For this review, take the finished solid that the model builds, in its own axes (mm). A direction names the side the tool comes from. Give positions to 0.01 mm unless a question says otherwise; leave off trailing zeros. Loops run counter-clockwise (first coordinate to the right, second up) from the corner with the lowest first, then second, coordinate; pieces in that order, holes last. Notation, with made-up numbers: (-35.75, 29) -> (17.25, 29) arc R28 cw to (17.25, 63) -> close; hole circle Ø8 at (34, 44). An arc over 180 degrees is marked (long way). Write each question's results on one line, items separated by ' | '. Start each with the question number.
```python
from build123d import *

# Parameters (mm, degrees)
SKETCH1_R           = 2.6
BOSS_EXTRUDE1_DEPTH = 5


with BuildPart() as part:
    # Sketch1 → Boss-Extrude1 (new body)
    with BuildSketch(Plane(origin=(0, 0, 0), x_dir=(1, 0, 0), z_dir=(0, 1, 0))):
        with BuildLine():
            Line((0.885, 8.705129235), (0.785, 9.969141137))
            Line((0.785, 9.969141137), (0.5, 10.988630488))
            ThreePointArc((0.5, 10.988630488), (0, 11), (-0.5, 10.988630488))
            Line((-0.5, 10.988630488), (-0.785, 9.969141137))
            Line((-0.785, 9.969141137), (-0.885, 8.705129235))
            ThreePointArc((-0.885, 8.705129235), (-1.368801569, 8.64227298), (-1.848347855, 8.552549924))
            Line((-1.848347855, 8.552549924), (-2.334054665, 9.72379498))
            Line((-2.334054665, 9.72379498), (-2.920145308, 10.605317128))
            ThreePointArc((-2.920145308, 10.605317128), (-3.399186938, 10.461621679), (-3.871201824, 10.296300134))
            Line((-3.871201824, 10.296300134), (-3.827213396, 9.238638299))
            Line((-3.827213396, 9.238638299), (-3.531717889, 8.005589844))
            ThreePointArc((-3.531717889, 8.005589844), (-3.972416873, 7.796307087), (-4.400766544, 7.562787438))
            Line((-4.400766544, 7.562787438), (-5.224635797, 8.526616022))
            Line((-5.224635797, 8.526616022), (-6.054446447, 9.183881436))
            ThreePointArc((-6.054446447, 9.183881436), (-6.465637775, 8.899186938), (-6.863463441, 8.596096183))
            Line((-6.863463441, 8.596096183), (-6.494792479, 7.603793176))
            Line((-6.494792479, 7.603793176), (-5.832726624, 6.522407541))
            ThreePointArc((-5.832726624, 6.522407541), (-6.187184335, 6.187184335), (-6.522407541, 5.832726624))
            Line((-6.522407541, 5.832726624), (-7.603793176, 6.494792479))
            Line((-7.603793176, 6.494792479), (-8.596096183, 6.863463441))
            ThreePointArc((-8.596096183, 6.863463441), (-8.899186938, 6.465637775), (-9.183881436, 6.054446447))
            Line((-9.183881436, 6.054446447), (-8.526616022, 5.224635797))
            Line((-8.526616022, 5.224635797), (-7.562787438, 4.400766544))
            ThreePointArc((-7.562787438, 4.400766544), (-7.796307087, 3.972416873), (-8.005589844, 3.531717889))
            Line((-8.005589844, 3.531717889), (-9.238638299, 3.827213396))
            Line((-9.238638299, 3.827213396), (-10.296300134, 3.871201824))
            ThreePointArc((-10.296300134, 3.871201824), (-10.461621679, 3.399186938), (-10.605317128, 2.920145308))
            Line((-10.605317128, 2.920145308), (-9.72379498, 2.334054665))
            Line((-9.72379498, 2.334054665), (-8.552549924, 1.848347855))
            ThreePointArc((-8.552549924, 1.848347855), (-8.64227298, 1.368801569), (-8.705129235, 0.885))
            Line((-8.705129235, 0.885), (-9.969141137, 0.785))
            Line((-9.969141137, 0.785), (-10.988630488, 0.5))
            ThreePointArc((-10.988630488, 0.5), (-11, 0), (-10.988630488, -0.5))
            Line((-10.988630488, -0.5), (-9.969141137, -0.785))
            Line((-9.969141137, -0.785), (-8.705129235, -0.885))
            ThreePointArc((-8.705129235, -0.885), (-8.64227298, -1.368801569), (-8.552549924, -1.848347855))
            Line((-8.552549924, -1.848347855), (-9.72379498, -2.334054665))
            Line((-9.72379498, -2.334054665), (-10.605317128, -2.920145308))
            ThreePointArc((-10.605317128, -2.920145308), (-10.461621679, -3.399186938), (-10.296300134, -3.871201824))
            Line((-10.296300134, -3.871201824), (-9.238638299, -3.827213396))
            Line((-9.238638299, -3.827213396), (-8.005589844, -3.531717889))
            ThreePointArc((-8.005589844, -3.531717889), (-7.796307087, -3.972416873), (-7.562787438, -4.400766544))
            Line((-7.562787438, -4.400766544), (-8.526616022, -5.224635797))
            Line((-8.526616022, -5.224635797), (-9.183881436, -6.054446447))
            ThreePointArc((-9.183881436, -6.054446447), (-8.899186938, -6.465637775), (-8.596096183, -6.863463441))
            Line((-8.596096183, -6.863463441), (-7.603793176, -6.494792479))
            Line((-7.603793176, -6.494792479), (-6.522407541, -5.832726624))
            ThreePointArc((-6.522407541, -5.832726624), (-6.187184335, -6.187184335), (-5.832726624, -6.522407541))
            Line((-5.832726624, -6.522407541), (-6.494792479, -7.603793176))
            Line((-6.494792479, -7.603793176), (-6.863463441, -8.596096183))
            ThreePointArc((-6.863463441, -8.596096183), (-6.465637775, -8.899186938), (-6.054446447, -9.183881436))
            Line((-6.054446447, -9.183881436), (-5.224635797, -8.526616022))
            Line((-5.224635797, -8.526616022), (-4.400766544, -7.562787438))
            ThreePointArc((-4.400766544, -7.562787438), (-3.972416873, -7.796307087), (-3.531717889, -8.005589844))
            Line((-3.531717889, -8.005589844), (-3.827213396, -9.238638299))
            Line((-3.827213396, -9.238638299), (-3.871201824, -10.296300134))
            ThreePointArc((-3.871201824, -10.296300134), (-3.399186938, -10.461621679), (-2.920145308, -10.605317128))
            Line((-2.920145308, -10.605317128), (-2.334054665, -9.72379498))
            Line((-2.334054665, -9.72379498), (-1.848347855, -8.552549924))
            ThreePointArc((-1.848347855, -8.552549924), (-1.368801569, -8.64227298), (-0.885, -8.705129235))
            Line((-0.885, -8.705129235), (-0.785, -9.969141137))
            Line((-0.785, -9.969141137), (-0.5, -10.988630488))
            ThreePointArc((-0.5, -10.988630488), (0, -11), (0.5, -10.988630488))
            Line((0.5, -10.988630488), (0.785, -9.969141137))
            Line((0.785, -9.969141137), (0.885, -8.705129235))
            ThreePointArc((0.885, -8.705129235), (1.368801569, -8.64227298), (1.848347855, -8.552549924))
            Line((1.848347855, -8.552549924), (2.334054665, -9.72379498))
            Line((2.334054665, -9.72379498), (2.920145308, -10.605317128))
            ThreePointArc((2.920145308, -10.605317128), (3.399186938, -10.461621679), (3.871201824, -10.296300134))
            Line((3.871201824, -10.296300134), (3.827213396, -9.238638299))
            Line((3.827213396, -9.238638299), (3.531717889, -8.005589844))
            ThreePointArc((3.531717889, -8.005589844), (3.972416873, -7.796307087), (4.400766544, -7.562787438))
            Line((4.400766544, -7.562787438), (5.224635797, -8.526616022))
            Line((5.224635797, -8.526616022), (6.054446447, -9.183881436))
            ThreePointArc((6.054446447, -9.183881436), (6.465637775, -8.899186938), (6.863463441, -8.596096183))
            Line((6.863463441, -8.596096183), (6.494792479, -7.603793176))
            Line((6.494792479, -7.603793176), (5.832726624, -6.522407541))
            ThreePointArc((5.832726624, -6.522407541), (6.187184335, -6.187184335), (6.522407541, -5.832726624))
            Line((6.522407541, -5.832726624), (7.603793176, -6.494792479))
            Line((7.603793176, -6.494792479), (8.596096183, -6.863463441))
            ThreePointArc((8.596096183, -6.863463441), (8.899186938, -6.465637775), (9.183881436, -6.054446447))
            Line((9.183881436, -6.054446447), (8.526616022, -5.224635797))
            Line((8.526616022, -5.224635797), (7.562787438, -4.400766544))
            ThreePointArc((7.562787438, -4.400766544), (7.796307087, -3.972416873), (8.005589844, -3.531717889))
            Line((8.005589844, -3.531717889), (9.238638299, -3.827213396))
            Line((9.238638299, -3.827213396), (10.296300134, -3.871201824))
            ThreePointArc((10.296300134, -3.871201824), (10.461621679, -3.399186938), (10.605317128, -2.920145308))
            Line((10.605317128, -2.920145308), (9.72379498, -2.334054665))
            Line((9.72379498, -2.334054665), (8.552549924, -1.848347855))
            ThreePointArc((8.552549924, -1.848347855), (8.64227298, -1.368801569), (8.705129235, -0.885))
            Line((8.705129235, -0.885), (9.969141137, -0.785))
            Line((9.969141137, -0.785), (10.988630488, -0.5))
            ThreePointArc((10.988630488, -0.5), (11, 0), (10.988630488, 0.5))
            Line((10.988630488, 0.5), (9.969141137, 0.785))
            Line((9.969141137, 0.785), (8.705129235, 0.885))
            ThreePointArc((8.705129235, 0.885), (8.64227298, 1.368801569), (8.552549924, 1.848347855))
            Line((8.552549924, 1.848347855), (9.72379498, 2.334054665))
            Line((9.72379498, 2.334054665), (10.605317128, 2.920145308))
            ThreePointArc((10.605317128, 2.920145308), (10.461621679, 3.399186938), (10.296300134, 3.871201824))
            Line((10.296300134, 3.871201824), (9.238638299, 3.827213396))
            Line((9.238638299, 3.827213396), (8.005589844, 3.531717889))
            ThreePointArc((8.005589844, 3.531717889), (7.796307087, 3.972416873), (7.562787438, 4.400766544))
            Line((7.562787438, 4.400766544), (8.526616022, 5.224635797))
            Line((8.526616022, 5.224635797), (9.183881436, 6.054446447))
            ThreePointArc((9.183881436, 6.054446447), (8.899186938, 6.465637775), (8.596096183, 6.863463441))
            Line((8.596096183, 6.863463441), (7.603793176, 6.494792479))
            Line((7.603793176, 6.494792479), (6.522407541, 5.832726624))
            ThreePointArc((6.522407541, 5.832726624), (6.187184335, 6.187184335), (5.832726624, 6.522407541))
            Line((5.832726624, 6.522407541), (6.494792479, 7.603793176))
            Line((6.494792479, 7.603793176), (6.863463441, 8.596096183))
            ThreePointArc((6.863463441, 8.596096183), (6.465637775, 8.899186938), (6.054446447, 9.183881436))
            Line((6.054446447, 9.183881436), (5.224635797, 8.526616022))
            Line((5.224635797, 8.526616022), (4.400766544, 7.562787438))
            ThreePointArc((4.400766544, 7.562787438), (3.972416873, 7.796307087), (3.531717889, 8.005589844))
            Line((3.531717889, 8.005589844), (3.827213396, 9.238638299))
            Line((3.827213396, 9.238638299), (3.871201824, 10.296300134))
            ThreePointArc((3.871201824, 10.296300134), (3.399186938, 10.461621679), (2.920145308, 10.605317128))
            Line((2.920145308, 10.605317128), (2.334054665, 9.72379498))
            Line((2.334054665, 9.72379498), (1.848347855, 8.552549924))
            ThreePointArc((1.848347855, 8.552549924), (1.368801569, 8.64227298), (0.885, 8.705129235))
        make_face()
        with Locations(Location((0, 0, 0), (0, 0, 270))):
            Circle(SKETCH1_R, mode=Mode.SUBTRACT)
    extrude(amount=BOSS_EXTRUDE1_DEPTH)


solid = part.part
```
1. Draft analysis for pull direction Z (two halves, no side actions). For faces 5 (the flat face through (3.85, 2.46, 9.77)), 6 (the flat face through (-9.346, 2.465, 0.834)), 7 (the flat face through (2.623, 2.465, 10.158)), 8 (the flat face through (0, 5, -3)), state which applies: released by +Z, released by -Z, zero draft, split by the parting line, or undercut.
2. We need section C-C (x = 5.5). Write out the cut boundary in (y, z), plus the area to 3 significant figures.
3. We need section B-B (z = 0). Write out the cut boundary in (x, y).
4. Wall thickness on L1, parallel to X at y = 0.8, z = -9; L2, parallel to Z at x = 9.75, y = 0.6; L3, parallel to Z at x = 7.75, y = 3.6: over which ranges is each line inside the solid? List them lowest first.
5. Machinability: for faces 1 (the flat face through (-8.093, 2.465, -6.677)), 2 (the flat face through (3.68, 2.46, 8.63)), 3 (the flat face through (2.088, 2.465, 9.13)), 4 (the flat face through (-10.472, 2.465, -0.644)), which of the approach directions +Z, -Z, +X, -X, +Y, -Y give a long, thin tool a straight path to every point of the face, cutting with its end or side? Answer none if there is none.
6. For pin 1 Ø2 at (x, z) = (-2.5, 5) entering from -Y; pin 2 Ø1.5 at (y, z) = (3, 7) entering from +X; pin 3 Ø1 at (x, y) = (3, 3) entering from -Z; pin 4 Ø1.5 at (y, z) = (1, -3.5) entering from +X, all flat-tipped, find the tip position at first contact; note any pin that passes through.
7. We need section A-A (x = 0). Write out the cut boundary in (y, z), plus the area to 3 significant figures.
Response:
1) face 5: undercut | face 6: undercut | face 7: released by +Z | face 8: zero draft
2) outline: (0, -8.74) -> (5, -8.74) -> (5, 8.74) -> (0, 8.74) -> close | area: 87.4 mm2
3) outline: (-11, 0) -> (-2.6, 0) -> (-2.6, 5) -> (-11, 5) -> close; (2.6, 0) -> (11, 0) -> (11, 5) -> (2.6, 5) -> close
4) L1: x = -6.32 to -5.82, -3.77 to -2.03, -0.86 to 0.86, 2.03 to 3.77, 5.82 to 6.32 | L2: z = -3.85 to -2.35, -0.8 to 0.8, 2.35 to 3.85 | L3: z = -6.55 to -4.56, -4.06 to 4.06, 4.56 to 6.55
5) face 1: -Z, +Y, -Y | face 2: +Y, -Y | face 3: +Z, +Y, -Y | face 4: -X, +Y, -Y
6) pin 1: stops at y = 0 | pin 2: stops at x = 9.05 | pin 3: stops at z = -10.61 | pin 4: stops at x = 10.61
7) outline: (0, -11) -> (5, -11) -> (5, -2.6) -> (0, -2.6) -> close; (0, 2.6) -> (5, 2.6) -> (5, 11) -> (0, 11) -> close | area: 84.0 mm2
